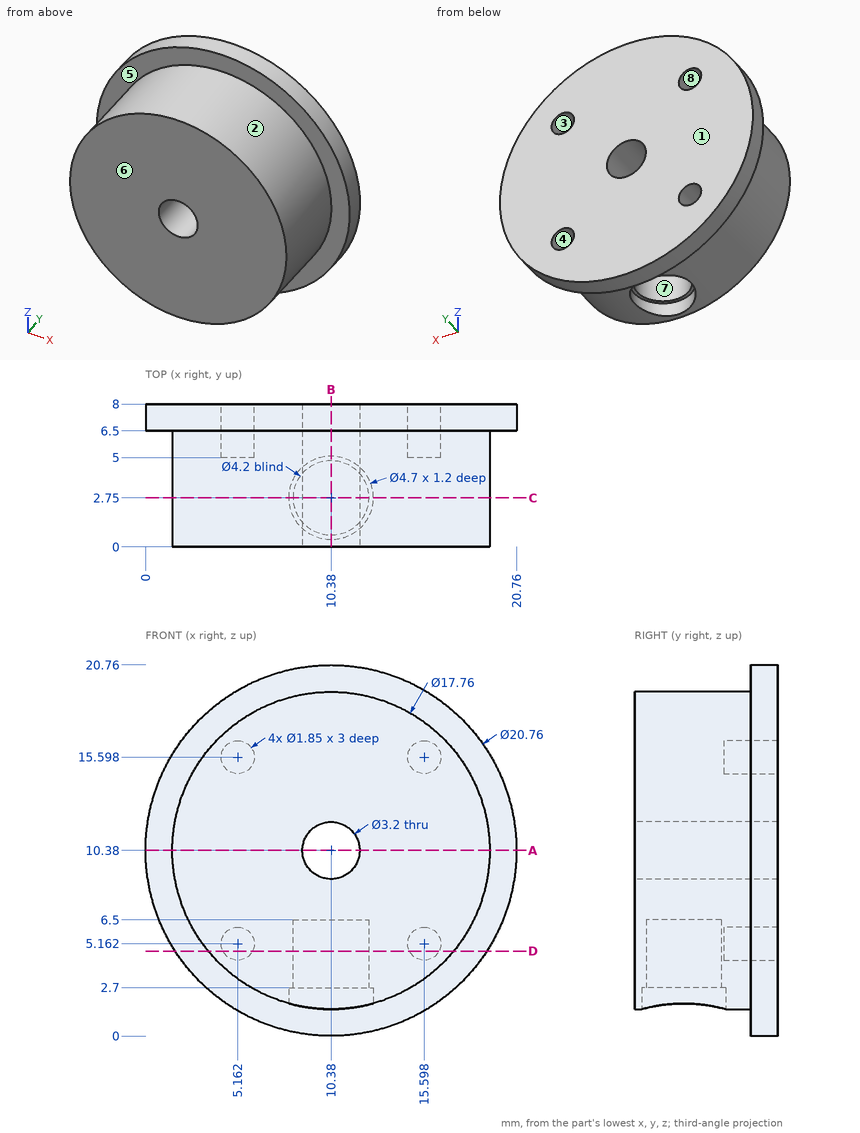
Could you check a few things on this drawing? It's one solid part, dimensions in mm from its lowest x, y, z. A direction names the side the tool comes from. Give positions to 0.01 mm unless a question says otherwise; leave off trailing zeros. Write each loop counter-clockwise with the first axis right and the second up, starting at its lowest first coordinate (ties: lowest second). Pieces come first, ordered by that corner, then holes. Notation, with made-up numbers: (-24.5, -18.75) -> (24.5, -18.75) arc R35 ccw to (24.5, 16.25) -> close; hole circle Ø10 at (81.25, -7). An arc over 180 degrees is marked (long way). Write each question's results on one line, items separated by ' | '.
1. I want a section at C-C, the plane y = 2.75. Write out the boundary of the cut face in (x, z), then the cut area to 3 significant figures.
Check sheet entries:
outline: (8.03, 1.82) -> (8.03, 2.7) -> (8.28, 2.7) -> (8.28, 6.5) -> (12.48, 6.5) -> (12.48, 2.7) -> (12.73, 2.7) -> (12.73, 1.82) arc R8.88 ccw (long way) to start; hole circle Ø3.2 at (10.38, 10.38) | area: 219 mm²
2. On a 3-axis mill with a long thin cutter (end or side, diameter ignored), from which of +Z, -Z, +X, -X, +Y, -Y can I reach the whole of each face in a straight line? I mean the marked faces 5, 6, 7 and 8. Say none if no direction works.
Check sheet entries:
face 5: -Y | face 6: +Z, -Z, +X, -X, -Y | face 7: -Z | face 8: +Y
3. I want a section at D-D, the plane z = 4.75. Write out the boundary of the cut face in (x, y).
Check sheet entries:
outline: (1.66, 6.5) -> (3.51, 6.5) -> (3.51, 0) -> (17.25, 0) -> (17.25, 6.5) -> (19.1, 6.5) -> (19.1, 8) -> (16.43, 8) -> (16.43, 5) -> (14.77, 5) -> (14.77, 8) -> (5.99, 8) -> (5.99, 5) -> (4.33, 5) -> (4.33, 8) -> (1.66, 8) -> close; hole circle Ø4.2 at (10.38, 2.75)
4. I need wall thicknesses on L1, parallel to Y at x = 10.38, z = 2.4; L2, parallel to X at y = 1, z = 10.5 (1 decimal); L3, parallel to Y at x = 10.38, z = 5.6. Which ranges of each line are inside material? Lowest first, please.
Check sheet entries:
L1: y = 0 to 0.4, 5.1 to 8 | L2: x = 1.5 to 8.8, 12 to 19.3 | L3: y = 0 to 0.65, 4.85 to 8
5. I want a section at A-A, the plane z = 10.38. Write out the boundary of the cut face in (x, y).
Check sheet entries:
outline: (0, 6.5) -> (1.5, 6.5) -> (1.5, 0) -> (8.78, 0) -> (8.78, 8) -> (0, 8) -> close; (11.98, 0) -> (19.26, 0) -> (19.26, 6.5) -> (20.76, 6.5) -> (20.76, 8) -> (11.98, 8) -> close
6. Will these pins go through, and if not, where does the flat tip stop? pin 1 Ø4 at (x, y) = (10.38, 2.75) entering from +Z; pin 2 Ø2 at (y, z) = (1, 13) entering from -X; pin 3 Ø1.1 at (x, z) = (5.16, 5.16) entering from +Y.
Check sheet entries:
pin 1: stops at z = 19.26 | pin 2: stops at x = 1.65 | pin 3: stops at y = 5
7. If we mould it in two halves opening along Z, with no side actions, what happens to the marked faces 1, 2, 3 and 4? For each: released by +Z, released by -Z, zero draft, split by the parting line, or undercut.
Check sheet entries:
face 1: zero draft | face 2: split by the parting line | face 3: undercut | face 4: undercut
8. I want a section at B-B, the plane x = 10.38. Write out the boundary of the cut face in (y, z).
Check sheet entries:
outline: (0, 1.5) -> (0.4, 1.5) -> (0.4, 2.7) -> (0.65, 2.7) -> (0.65, 6.5) -> (4.85, 6.5) -> (4.85, 2.7) -> (5.1, 2.7) -> (5.1, 1.5) -> (6.5, 1.5) -> (6.5, 0) -> (8, 0) -> (8, 8.78) -> (0, 8.78) -> close; (0, 11.98) -> (8, 11.98) -> (8, 20.76) -> (6.5, 20.76) -> (6.5, 19.26) -> (0, 19.26) -> close
